Build history of the part. All positions in model axes, mm. Face numbers are marked on the shaded views. A direction names the side the tool comes from. Give positions to 0.01 mm unless a question says otherwise; leave off trailing zeros. Loops run counter-clockwise (first coordinate to the right, second up) from the corner with the lowest first, then second, coordinate; pieces in that order, holes last. Notation, with made-up numbers: (-38, 55.25) - (-10, 55.25) arc R27 ccw to (-10, 87.25) - close; hole circle Ø10 at (-27.5, 34.5). An arc over 180 degrees is marked (long way). Return JSON: item names as keys, results as strings. Group by question number.
1) Slice it at A-A (y = 14). List the corners of the cut face in (x, z) (3 decimals), and give its area (3 significant figures).
2) Slice it at B-B (z = 0). List the corners of the cut face in (x, y) (3 decimals), and give its area (3 significant figures).
3) Slice it at D-D (x = -16.5). List the corners of the cut face in (y, z) (3 decimals), and give its area (3 significant figures).
4) Mould opens along X. For the marked faces 1, 2, 3 and 4 say: released by +X, released by -X, zero draft, split by the parting line, or undercut.
5) Drop flat-ended pins along their axis: pin 1 (1 mm diameter, centred on y = 18.5, z = 4, fed in from +X); pin 2 (1 mm diameter, centred on y = 17, z = 0, fed in from -X); pin 3 (5 mm diameter, centred on x = 11, z = -3.5, fed in from +Y). Give the stop position or say it passes through.
6) 3-axis set-ups, long thin cutter, end or side, ignore diameter. For the marked faces 5, 6 and 7: which of +Z, -Z, +X, -X, +Y, -Y reach the whole face in a straight line?
7) Drill centre lines: probe 1 along Z at (x, y) = (16.5, 8.5) (3 decimals); probe 2 along Y at (x, z) = (3.5, 0.25) (3 decimals); probe 3 along X at (y, z) = (1.75, -2). Where is each one in solid material? Low to high. Write a range as from..to.
8) Slice it at C-C (x = -1). List the corners of the cut face in (y, z) (3 decimals).
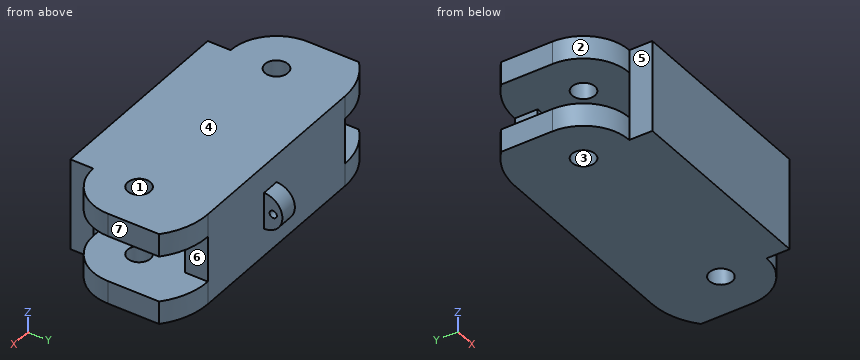
```python
from build123d import *

# Parameters (mm, degrees)
SKETCH1_W           = 47.625
SKETCH1_H           = 19.05
BOSS_EXTRUDE1_DEPTH = 19.05
SKETCH2_R           = 1.5875
CUT_EXTRUDE1_DEPTH  = 19.05
SKETCH9_W           = 2.54
SKETCH9_H           = 5.08
BOSS_EXTRUDE2_DEPTH = 2.54
SKETCH3_R           = 0.508
SKETCH3_W           = 6.35
SKETCH3_H           = 12.7
CUT_EXTRUDE2_DEPTH  = 38.1
SKETCH4_W           = 15.197967332
SKETCH4_H           = 6.35
CUT_EXTRUDE3_DEPTH  = 43.18
CUT_EXTRUDE4_DEPTH  = 19.05
SKETCH7_W           = 13.77890267
SKETCH7_H           = 6.35
CUT_EXTRUDE5_DEPTH  = 3.81


with BuildPart() as part:
    # Sketch1 → Boss-Extrude1 (new body)
    with BuildSketch(Plane(origin=(0, 0, 0), x_dir=(1, 0, 0), z_dir=(0, 1, 0))):
        with Locations((0.3175, 0)):
            Rectangle(SKETCH1_W, SKETCH1_H)
    extrude(amount=BOSS_EXTRUDE1_DEPTH)

    # Sketch2 → Cut-Extrude1 (cut)
    with BuildSketch(Plane.XY.offset(9.525)):
        with Locations((-13.97, 9.525)):
            Circle(SKETCH2_R)
        with Locations((13.97, 9.525)):
            Circle(SKETCH2_R)
        with BuildLine():
            ThreePointArc((-13.97, 19.05), (-23.495, 9.525), (-13.97, 0))
            ThreePointArc((-13.97, 0), (-34.184765451, 9.525), (-13.97, 19.05))
        make_face()
        with BuildLine():
            ThreePointArc((13.97, 19.05), (34.184765451, 9.525), (13.97, 0))
            ThreePointArc((13.97, 0), (23.495, 9.525), (13.97, 19.05))
        make_face()
    extrude(amount=-CUT_EXTRUDE1_DEPTH, mode=Mode.SUBTRACT)

    # Sketch9 → Boss-Extrude2 (add)
    with BuildSketch(Plane(origin=(0, 19.05, 0), x_dir=(1, 0, 0), z_dir=(0, 1, 0))):
        with Locations((1.27, 0)):
            Rectangle(SKETCH9_W, SKETCH9_H)
    extrude(amount=BOSS_EXTRUDE2_DEPTH)

    # Sketch3 → Cut-Extrude2 (cut, symmetric)
    with BuildSketch(Plane(origin=(0, 0, 0), x_dir=(0, 0, -1), z_dir=(1, 0, 0))):
        with Locations((0, 20.32)):
            Circle(SKETCH3_R)
        with Locations((0, 9.525)):
            Rectangle(SKETCH3_W, SKETCH3_H)
        with BuildLine():
            ThreePointArc((-2.54, 19.05), (0, 21.59), (2.54, 19.05))
            ThreePointArc((2.54, 19.05), (0, 24.1080653), (-2.54, 19.05))
        make_face()
    extrude(amount=CUT_EXTRUDE2_DEPTH, both=True, mode=Mode.SUBTRACT)

    # Sketch4 → Cut-Extrude3 (cut)
    with BuildSketch(Plane(origin=(0, 19.05, 0), x_dir=(1, 0, 0), z_dir=(0, 1, 0))):
        Polygon((-29.361154188, -9.525), (-13.97, -9.525), (1.5875, -9.525), (28.406626571, -9.525), (28.406626571, -6.35), (1.5875, -6.35), (-13.97, -6.35), (-29.361154188, -6.35), align=None)
        Polygon((-13.97, 6.35), (-31.510324581, 6.35), (-31.510324581, 9.525), (-11.1125, 9.525), (1.5875, 9.525), (30.675017081, 9.525), (30.675017081, 6.35), (1.5875, 6.35), align=None)
        with Locations((21.568983666, 0)):
            Rectangle(SKETCH4_W, SKETCH4_H)
    extrude(amount=-CUT_EXTRUDE3_DEPTH, mode=Mode.SUBTRACT)

    # Sketch6 → Cut-Extrude4 (cut)
    with BuildSketch(Plane.XY.offset(9.525)):
        with BuildLine():
            Line((13.97, 0), (31.980086248, 0))
            Line((31.980086248, 0), (31.980086248, 3.175))
            Line((31.980086248, 3.175), (27.183594801, 13.808491056))
            Line((27.183594801, 13.808491056), (20.32, 24.370653281))
            Line((20.32, 24.370653281), (20.32, 9.525))
            ThreePointArc((20.32, 9.525), (18.460128061, 5.034871939), (13.97, 3.175))
            Line((13.97, 3.175), (13.97, 0))
        make_face()
        with BuildLine():
            Line((-13.97, 0), (-13.97, 3.175))
            ThreePointArc((-13.97, 3.175), (-18.460128061, 5.034871939), (-20.32, 9.525))
            Line((-20.32, 9.525), (-20.32, 20.942771878))
            Line((-20.32, 20.942771878), (-28.921644245, 11.767684684))
            Line((-28.921644245, 11.767684684), (-28.921644245, 0))
            Line((-28.921644245, 0), (-13.97, 0))
        make_face()
    extrude(amount=-CUT_EXTRUDE4_DEPTH, mode=Mode.SUBTRACT)

    # Sketch7 → Cut-Extrude5 (cut)
    with BuildSketch(Plane(origin=(0, 19.05, 0), x_dir=(1, 0, 0), z_dir=(0, 1, 0))):
        with Locations((-20.859451335, 0)):
            Rectangle(SKETCH7_W, SKETCH7_H)
    extrude(amount=-CUT_EXTRUDE5_DEPTH, mode=Mode.SUBTRACT)


solid = part.part
```
Results:
{
 "1": {"outline": "(-20.32, -6.35) - (20.32, -6.35) - (20.32, -3.175) - (-20.32, -3.175) - close; (-20.32, 3.175) - (20.32, 3.175) - (20.32, 6.35) - (-20.32, 6.35) - close", "area": "258 mm2"},
 "2": {"outline": "(-13.97, 0) - (13.97, 0) - (13.97, 3.175) - (-13.97, 3.175) - close; (-13.97, 15.875) - (13.97, 15.875) - (13.97, 19.05) - (2.54, 19.05) - (2.54, 19.812) - (0, 19.812) - (0, 19.05) - (-13.97, 19.05) - close; (0, 20.828) - (2.54, 20.828) - (2.54, 21.59) - (0, 21.59) - close", "area": "181 mm2"},
 "3": {"outline": "(3.701, -6.35) - (18.708, -6.35) - (18.708, -3.175) - (3.701, -3.175) - close; (3.701, 3.175) - (18.708, 3.175) - (18.708, 6.35) - (3.701, 6.35) - close", "area": "95.3 mm2"},
 "4": {"face 1": "undercut", "face 2": "released by -X", "face 3": "undercut", "face 4": "zero draft"},
 "5": {"pin 1": "x = 18.32", "pin 2": "x = -13.97", "pin 3": "y = 19.05"},
 "6": {"face 5": "+Z, -Z, -X, -Y", "face 6": "+X, +Y, -Y", "face 7": "+Z, -Z, +X, +Y, -Y"},
 "7": {"probe 1": "-6.35..-3.175, 3.175..6.35", "probe 2": "0..3.175, 15.875..19.05", "probe 3": "-13.97..13.97"},
 "8": {"outline": "(0, -6.35) - (19.05, -6.35) - (19.05, 6.35) - (0, 6.35) - close; hole (3.175, -3.175) - (15.875, -3.175) - (15.875, 3.175) - (3.175, 3.175) - close"}
}
